```python
from build123d import *

# Parameters (mm, degrees)
F0_R            = 2.5
F0_R_2          = 1.15
F1_DEPTH        = 1
F2_W            = 15
F2_H            = 15
F2_R            = 5
F2_R_2          = 2.5
F2_R_3          = 1.15
F3_DEPTH        = 1
F4_R            = 3
F5_R            = 0.75
F6_DEPTH        = 25
F6_COPIES_COUNT = 4


# Not quite as in the source:
# - a pattern or mirror of a feature is missing from the dataset's text; its kind, count and spacing are read off the source's solid


with BuildPart() as f1:
    # F0 (on Top) → F1 (new body)
    with BuildSketch(Plane.XY):
        Circle(F0_R)
        Circle(F0_R_2, mode=Mode.SUBTRACT)
    extrude(amount=F1_DEPTH)

    # F2 (on face) → F3 (join)
    with BuildSketch(Plane(origin=(0, 0, 0), x_dir=(1, 0, 0), z_dir=(0, 0, -1))):
        Rectangle(F2_W, F2_H)
        Circle(F2_R, mode=Mode.SUBTRACT)
        Circle(F2_R)
        Circle(F2_R_2, mode=Mode.SUBTRACT)
        Circle(F2_R_2)
        Circle(F2_R_3, mode=Mode.SUBTRACT)
    extrude(amount=F3_DEPTH)

    # F4
    f4_edges = [f1.edges().sort_by_distance(p)[0] for p in [
        (-7.5, 7.5, -0.5),
        (7.5, 7.5, -0.5),
        (-7.5, -7.5, -0.5),
        (7.5, -7.5, -0.5),
    ]]
    fillet(f4_edges, radius=F4_R)

    # F5 (on face) → F6 (cut)
    with BuildSketch(Plane.XY):
        with Locations((-4.5, 4.5)):
            Circle(F5_R)
        with Locations((-1.5, 4.5)):
            Circle(F5_R)
    f6 = extrude(amount=-F6_DEPTH, mode=Mode.SUBTRACT)

    # F6_copies: F6 ×4 about axis
    f6_copies_axis = Axis((0, 0, 0), (0, 0, 1))
    for i in range(1, F6_COPIES_COUNT):
        add(f6.rotate(f6_copies_axis, i * 360 / F6_COPIES_COUNT), mode=Mode.SUBTRACT)


solid = f1.part
```
Source: CAD feature listing. Evaluate the final solid. Frame: model axes, mm. A direction names the side the tool comes from. Give positions to 0.01 mm unless a question says otherwise; leave off trailing zeros. Write each loop counter-clockwise with the first axis right and the second up, starting at its lowest first coordinate (ties: lowest second). Pieces come first, ordered by that corner, then holes. Notation, with made-up numbers: (48, 10.5) - (60, 10.5) arc R26 cw to (60, 42.5) - close; hole circle Ø3 at (-11, 21). An arc over 180 degrees is marked (long way). One line per item, written item: value. Start each with the question number.
Q1. First-contact query: pin 1 Ø2.5 at (x, y) = (-1.5, 4.5) entering from +Z. Flat tip, straight axial feed; report the tip coordinate or a pass-through.
Q2. Set-up query: faces 1 (the face through (-3.768, -1.663, -0.493)), 2 (the face through (-0.54, -2.44, 0.49)). Return all of +Z, -Z, +X, -X, +Y, -Y with unobstructed straight access to the full face (end or side cutting, diameter ignored); none if empty.
Q3. Section query C-C, the plane z = -0.65. Count the separate pieces of the cut face and the enclosed holes in it, then the cut area to 3 significant figures.
Q4. Section query D-D, the plane y = 4.25. Return the cut outline in (x, z), then the cut area to 3 significant figures.
Q5. Material intervals for probe 1 along X at (y, z) = (-4.5, -0.45); probe 2 along Z at (x, y) = (-6, -2); probe 3 along Y at (x, z) = (-0.5, 0.65), sorted ascending. Write a range as from..to.
Q6. Section query B-B, the plane x = 0. Return the cut outline in (y, z), then the cut area to 3 significant figures.
Q7. Draft query along Y for faces 3 (the face through (1, -1, 1)), 4 (the face through (-0.91, 0.7, 0.01)), 5 (the face through (-0.1, -7.5, -0.5)). Return one class per face: +Y half, -Y half, draft (parallel to the pull), parting line (faces both ways), or undercut.
Q8. Section query A-A, the plane y = -1.5. Return the cut outline in (x, z), then the cut area to 3 significant figures.
Answer:
1. pin 1: stops at z = 0
2. face 1: +Z, -Z
2. face 2: +Z
3. separate pieces: 1
3. enclosed holes: 9
3. area: 199 mm2
4. outline: (-7.5, -1) - (-5.21, -1) - (-5.21, 0) - (-7.5, 0) - close; (-3.79, -1) - (-2.21, -1) - (-2.21, 0) - (-3.79, 0) - close; (-0.79, -1) - (3.79, -1) - (3.79, 0) - (-0.79, 0) - close; (5.21, -1) - (7.5, -1) - (7.5, 0) - (5.21, 0) - close
4. area: 10.8 mm2
5. probe 1: x = -7.5..-5.25, -3.75..0.75, 2.25..3.75, 5.25..7.5
5. probe 2: z = -1..0
5. probe 3: y = -2.45..-1.04, 1.04..2.45
6. outline: (-7.5, -1) - (-1.15, -1) - (-1.15, 1) - (-2.5, 1) - (-2.5, 0) - (-7.5, 0) - close; (1.15, -1) - (7.5, -1) - (7.5, 0) - (2.5, 0) - (2.5, 1) - (1.15, 1) - close
6. area: 15.4 mm2
7. face 3: draft
7. face 4: undercut
7. face 5: -Y half
8. outline: (-7.5, -1) - (-5.25, -1) - (-5.25, 0) - (-7.5, 0) - close; (-3.75, -1) - (7.5, -1) - (7.5, 0) - (2, 0) - (2, 1) - (-2, 1) - (-2, 0) - (-3.75, 0) - close
8. area: 17.5 mm2
